Read the model definition and answer for the solid it produces. Units are mm, in the model's axes. A direction names the side the tool comes from. Give positions to 0.01 mm unless a question says otherwise; leave off trailing zeros. Loops run counter-clockwise (first coordinate to the right, second up) from the corner with the lowest first, then second, coordinate; pieces in that order, holes last. Notation, with made-up numbers: M 71,14.25 L 128,14.25 A18 cw 128,29.25 Z; hole C 40,4.25 d10. An arc over 180 degrees is marked long. Return JSON: item names as keys, results as strings. Group by question number.
```python
from build123d import *

# Parameters (mm, degrees)
F0_W     = 50
F0_H     = 40
F1_DEPTH = 50
F2_R     = 17.5
F3_DEPTH = 34
F4_R     = 8
F5_DEPTH = 84.001


with BuildPart() as f1:
    # F0 (on Top) → F1 (new body)
    with BuildSketch(Plane.XY):
        Rectangle(F0_W, F0_H)
    extrude(amount=F1_DEPTH)

    # F2 (on face) → F3 (join)
    with BuildSketch(Plane(origin=(0, 0, 0), x_dir=(1, 0, 0), z_dir=(0, 0, -1))):
        Circle(F2_R)
    extrude(amount=F3_DEPTH)

    # F4 (on face) → F5 (cut, through all)
    with BuildSketch(Plane.XY.offset(50)):
        Circle(F4_R)
    extrude(amount=-F5_DEPTH, mode=Mode.SUBTRACT)


solid = f1.part
```
1. Find section D-D (y = 14). Write down the section's boundary in (x, z).
2. Find section C-C (z = 45.5). Write down the section's boundary in (x, y), and give its area (3 significant figures).
3. Straight lines are drawn through the part: line 1 along Y through (x, z) = (0, 27); line 2 along Y through (x, z) = (0, -15); line 3 along Z through (x, y) = (-16, 13.5). For each, find the intervals that lie inside material, in ascending order.
4. Find section A-A (y = 0). Write down the section's boundary in (x, z).
5. The mould has two halves that part along X. Classify faces 1 (the cylindrical face through (-1.73, -7.81, 8.59)), 2 (the flat face through (-25, 0, 25)), 3 (the flat face through (-17, 5, 0)): +X half, -X half, draft (parallel to the pull), parting line (faces both ways), or undercut.
6. Find section B-B (x = 0). Write down the section's boundary in (y, z), and give its area (3 significant figures).
7. Flat-ended cylindrical pins translate along their axes: P1, Ø14.5, axis at x = 0, y = 0, coming from the -Z side; P2, Ø12, axis at x = 0.5, z = -25, coming from the +Y side; P3, Ø5, axis at x = 14.5, y = -11.5, coming from the -Z side. Find the tip coordinate at first contact, or state that the pin passes through.
8. For faces 4 (the flat face through (25, 0, 25)), 5 (the cylindrical face through (-13.887, 10.648, -16.762)), determine the directions among +Z, -Z, +X, -X, +Y, -Y from which every point of the face is accessible in a straight line to the end or side of a thin tool.
Result:
{
 "1": {"outline": "M -25,0 L -10.5,0 L -10.5,-34 L 10.5,-34 L 10.5,0 L 25,0 L 25,50 L -25,50 Z"},
 "2": {"outline": "M -25,-20 L 25,-20 L 25,20 L -25,20 Z; hole C 0,0 d16", "area": "1,800 mm2"},
 "3": {"line 1": "y = -20 to -8, 8 to 20", "line 2": "y = -17.5 to -8, 8 to 17.5", "line 3": "z = 0 to 50"},
 "4": {"outline": "M -25,0 L -17.5,0 L -17.5,-34 L -8,-34 L -8,50 L -25,50 Z; M 8,-34 L 17.5,-34 L 17.5,0 L 25,0 L 25,50 L 8,50 Z"},
 "5": {"face 1": "undercut", "face 2": "-X half", "face 3": "draft"},
 "6": {"outline": "M -20,0 L -17.5,0 L -17.5,-34 L -8,-34 L -8,50 L -20,50 Z; M 8,-34 L 17.5,-34 L 17.5,0 L 20,0 L 20,50 L 8,50 Z", "area": "1,850 mm2"},
 "7": {"P1": "passes through", "P2": "stops at y = 17.5", "P3": "stops at z = -34"},
 "8": {"face 4": "+Z, -Z, +X, +Y, -Y", "face 5": "-Z"}
}
